The model under review builds one solid part; all positions refer to its coordinate system, in mm. A direction names the side the tool comes from. Coordinates: 2 decimals unless noted, no trailing zeros. Loops run counter-clockwise (first coordinate to the right, second up) from the corner with the lowest first, then second, coordinate; pieces in that order, holes last. Notation, with made-up numbers: M 85,-25 L 136,-25 A18 cw 136,-16 Z; hole C 85.25,85 d2. An arc over 180 degrees is marked long. One line per item, written item: value.
```python
from build123d import *

# Parameters (mm, degrees)
SKETCH4_R                = 2.25
CUT_4XD4_5_PCD67_5_DEPTH = 150


with BuildPart() as part:
    # Sketch3 → REV_Seal_Cover_28x42x7 (revolve)
    with BuildSketch(Plane(origin=(0, 0, 0), x_dir=(1, 0, 0), z_dir=(0, 1, 0))):
        Polygon((15, 105), (40, 105), (40, 96), (27.5, 96), (27.5, 93), (24, 93), (24, 97), (21, 97), (21, 104), (15, 104), align=None)
    revolve(axis=Axis((0, 0, 150), (0, 0, -1)))

    # Sketch4 → CUT_4xD4.5_PCD67.5 (cut, symmetric)
    with BuildSketch(Plane.XY):
        with Locations(Location((23.8649, 23.8649, 0), (0, 0, 180))):
            Circle(SKETCH4_R)
        with Locations(Location((-23.8649, 23.8649, 0), (0, 0, 180))):
            Circle(SKETCH4_R)
        with Locations(Location((-23.8649, -23.8649, 0), (0, 0, 180))):
            Circle(SKETCH4_R)
        with Locations(Location((23.8649, -23.8649, 0), (0, 0, 180))):
            Circle(SKETCH4_R)
    extrude(amount=CUT_4XD4_5_PCD67_5_DEPTH, both=True, mode=Mode.SUBTRACT)


solid = part.part
```
(1) Tool access review of faces 4 (the face through (-8, -23, -93)), 5 (the face through (20.03, -6.31, -100.55)): name each direction out of +Z, -Z, +X, -X, +Y, -Y from which nothing blocks a thin tool from reaching the whole face with its end or side.
Checks:
face 4: +Z, +X, -X, +Y, -Y
face 5: +Z
(2) Add section C-C on y = 20. State the section outline as (x, z) points.
Checks:
outline: M -34.64,-105 L 34.64,-105 L 34.64,-96 L 18.87,-96 L 18.87,-93 L 13.27,-93 L 13.27,-97 L 6.4,-97 L 6.4,-104 L -6.4,-104 L -6.4,-97 L -13.27,-97 L -13.27,-93 L -18.87,-93 L -18.87,-96 L -34.64,-96 Z
(3) Insertion check: pin 1 Ø7 at (x, y) = (-23.86, 23.86) entering from -Z; pin 2 Ø2.5 at (x, y) = (23.86, -23.86) entering from -Z; pin 3 Ø6 at (x, z) = (8.5, -102) entering from +Y; pin 4 Ø1.5 at (x, z) = (25.5, -100) entering from -Y. Each pin has a flat end and moves straight along its axis. Give the tip position at first contact, or say it passes through.
Checks:
pin 1: z = -105
pin 2: through
pin 3: y = 39.62
pin 4: y = -31.42
(4) Draft analysis for pull direction Y (two halves, no side actions). For faces 1 (the face through (-5.961, 26.846, -94.479)), 2 (the face through (26.1, -9.4, -96)), 3 (the face through (-24.903, -21.869, -100.437)), state which applies: pulls with the +Y half, pulls with the -Y half, needs draft (parallel to the pull), parting line crosses it, or undercut.
Checks:
face 1: parting line crosses it
face 2: needs draft
face 3: undercut
(5) To check wall thickness, follow L1, parallel to Y at x = -1, z = -93.5; L2, parallel to X at y = 0, z = -104.7; L3, parallel to X at y = 0, z = -102. State the ranges of each line that lie inside material, in increasing order. Write a range as [from, to].
Checks:
L1: [-27.48, -23.98], [23.98, 27.48]
L2: [-40, -15], [15, 40]
L3: [-40, -21], [21, 40]
(6) Add section A-A on y = 0. State the section outline as (x, z) points.
Checks:
outline: M -40,-105 L -15,-105 L -15,-104 L -21,-104 L -21,-97 L -24,-97 L -24,-93 L -27.5,-93 L -27.5,-96 L -40,-96 Z; M 15,-105 L 40,-105 L 40,-96 L 27.5,-96 L 27.5,-93 L 24,-93 L 24,-97 L 21,-97 L 21,-104 L 15,-104 Z
(7) Add section D-D on x = -18.5. State the section outline as (y, z) points, then the cut area to 3 significant figures.
Checks:
outline: M -35.46,-105 L 35.46,-105 L 35.46,-96 L 20.35,-96 L 20.35,-93 L 15.29,-93 L 15.29,-97 L 9.94,-97 L 9.94,-104 L -9.94,-104 L -9.94,-97 L -15.29,-97 L -15.29,-93 L -20.35,-93 L -20.35,-96 L -35.46,-96 Z
area: 499 mm^2
